Could you check a few things on this model? Use its own coordinates, in mm. Give positions to 0.01 mm unless a question says otherwise; leave off trailing zeros. Loops run counter-clockwise (first coordinate to the right, second up) from the corner with the lowest first, then second, coordinate; pieces in that order, holes last. Notation, with made-up numbers: (1.5, 21) - (52.5, 21) arc R21 ccw to (52.5, 57) - close; hole circle Ø7 at (-21, 12). An arc over 180 degrees is marked (long way). One line per item, written item: value. Start each with the question number.
Q1. I want a section at B-B (z = 10.25). Please give me the cut outline in (x, y).
Q2. I want a section at A-A (z = 3.25). Please give me the cut outline in (x, y), then the cut area to 3 significant figures.
Q3. If we mould it in two halves opening along Z, with no side actions, what happens to faces 1 (the face through (12, -39, 14)), 2 (the face through (40, -14, 5)), 3 (the face through (20, -39, 0))? For each: released by +Z, released by -Z, zero draft, split by the parting line, or undercut.
Q4. If I drill on line 1 (Y direction, x = 25, z = 8); line 2 (Y direction, x = 21, z = 9); line 3 (X direction, y = -7.5, z = 12.25), over which ranges is the centre line in solid material (lowest first)? Write a range as from..to.
```python
from build123d import *

# Parameters (mm, degrees)
F0_W         = 40
F0_H         = 80
F1_DEPTH     = 14
F4_T1_DEPTH  = 17.8405087492
F4_T3_DEPTH  = 17.8405087492
F4_T5_DEPTH  = 36
F4_T7_DEPTH  = 76
F4_T9_DEPTH  = 17
F4_S13_W     = 2
F4_S13_H     = 2
F4_T14_DEPTH = 2
F4_S19_W     = 2
F4_S19_H     = 2
F4_T20_DEPTH = 2
F4_S25_W     = 2
F4_S25_H     = 2
F4_T26_DEPTH = 2
F4_S31_W     = 2
F4_S31_H     = 2
F4_T32_DEPTH = 2
F4_T36_ANGLE = 193.2912055484


# Not quite as in the source:
# - a fillet or chamfer that OpenCascade refuses, or shapes differently, is made with other operations: its cross-section is extruded or revolved along the edge and cut away or added


with BuildPart() as f1:
    # F0 (on Top) → F1 (new body)
    with BuildSketch(Plane.XY):
        with Locations((20, -40)):
            Rectangle(F0_W, F0_H)
    extrude(amount=F1_DEPTH)

    # F2 (on face) → F3 (revolve, cut)
    with BuildSketch(Plane.YZ.offset(40)):
        with BuildLine():
            Line((-40, 0), (-32.5033340744, 0))
            ThreePointArc((-32.5033340744, 0), (-22.2346925053, 5.186748348), (-14.8405087492, 14))
            Line((-14.8405087492, 14), (-40, 14))
            Line((-40, 14), (-40, 0))
        make_face()
        with BuildLine():
            Line((-40, 14), (-14.8405087492, 14))
            ThreePointArc((-14.8405087492, 14), (-15.4345771459, 42.2458185159), (-40, 56.2))
            Line((-40, 56.2), (-40, 14))
        make_face()
        with BuildLine():
            Line((-40, 0), (-40, -1))
            ThreePointArc((-40, -1), (-36.2184659198, -0.7488976858), (-32.5033340744, 0))
            Line((-32.5033340744, 0), (-40, 0))
        make_face()
    revolve(axis=Axis((40, -40, 27.6), (0, 0, -1)), mode=Mode.SUBTRACT)

    # F4: fillet of radius 2 on 10 edges, made by hand

    # F4_s2 → F4_t1 (cut)
    with BuildSketch(Plane.XZ.offset(2)):
        with BuildLine():
            ThreePointArc((40, 12), (39.4142135624, 13.4142135624), (38, 14))
            Line((38, 14), (40, 14))
            Line((40, 14), (40, 12))
        make_face()
    extrude(amount=F4_T1_DEPTH, mode=Mode.SUBTRACT)

    # F4_s4 → F4_t3 (cut)
    with BuildSketch(Plane.XZ.offset(60.1594912508)):
        with BuildLine():
            ThreePointArc((38, 14), (39.4142135624, 13.4142135624), (40, 12))
            Line((40, 12), (40, 14))
            Line((40, 14), (38, 14))
        make_face()
    extrude(amount=F4_T3_DEPTH, mode=Mode.SUBTRACT)

    # F4_s6 → F4_t5 (cut)
    with BuildSketch(Plane.YZ.offset(2)):
        with BuildLine():
            ThreePointArc((-78, 14), (-79.4142135624, 13.4142135624), (-80, 12))
            Line((-80, 12), (-80, 14))
            Line((-80, 14), (-78, 14))
        make_face()
        with BuildLine():
            ThreePointArc((0, 12), (-0.5857864376, 13.4142135624), (-2, 14))
            Line((-2, 14), (0, 14))
            Line((0, 14), (0, 12))
        make_face()
    extrude(amount=F4_T5_DEPTH, mode=Mode.SUBTRACT)

    # F4_s8 → F4_t7 (cut)
    with BuildSketch(Plane.XZ.offset(2)):
        with BuildLine():
            ThreePointArc((0, 12), (0.5857864376, 13.4142135624), (2, 14))
            Line((2, 14), (0, 14))
            Line((0, 14), (0, 12))
        make_face()
    extrude(amount=F4_T7_DEPTH, mode=Mode.SUBTRACT)

    # F4_s10 → F4_t9 (cut)
    with BuildSketch(Plane.XY.offset(-5)):
        with BuildLine():
            ThreePointArc((38, -80), (39.4142135624, -79.4142135624), (40, -78))
            Line((40, -78), (40, -80))
            Line((40, -80), (38, -80))
        make_face()
        with BuildLine():
            ThreePointArc((0, -78), (0.5857864376, -79.4142135624), (2, -80))
            Line((2, -80), (0, -80))
            Line((0, -80), (0, -78))
        make_face()
        with BuildLine():
            ThreePointArc((38, 0), (39.4142135624, -0.5857864376), (40, -2))
            Line((40, -2), (40, 0))
            Line((40, 0), (38, 0))
        make_face()
        with BuildLine():
            ThreePointArc((2, 0), (0.5857864376, -0.5857864376), (0, -2))
            Line((0, -2), (0, 0))
            Line((0, 0), (2, 0))
        make_face()
    extrude(amount=F4_T9_DEPTH, mode=Mode.SUBTRACT)


with BuildPart() as f4_tool12:
    # F4_s13 → F4_t14 (new body)
    with BuildSketch(Plane.XZ.offset(2)):
        with Locations((39, 13)):
            Rectangle(F4_S13_W, F4_S13_H)
    extrude(amount=-F4_T14_DEPTH)

    # F4_s15 → F4_t16 (revolve, cut)
    with BuildSketch(Plane(origin=(38, -2, 12), x_dir=(-0.7071067812, 0, -0.7071067812), z_dir=(0.7071067812, 0, -0.7071067812))):
        with BuildLine():
            ThreePointArc((0, -2), (2, 0), (0, 2))
            Line((0, 2), (0, -2))
        make_face()
    revolve(axis=Axis((38, -2, 12), (0, 1, 0)), mode=Mode.SUBTRACT)


with BuildPart() as f1_1:
    add(f1.part)

    # F4_t11: cut F4_tool12
    add(f4_tool12.part, mode=Mode.SUBTRACT)


with BuildPart() as f4_tool18:
    # F4_s19 → F4_t20 (new body)
    with BuildSketch(Plane.XY.offset(12)):
        with Locations((39, -79)):
            Rectangle(F4_S19_W, F4_S19_H)
    extrude(amount=F4_T20_DEPTH)

    # F4_s21 → F4_t22 (revolve, cut)
    with BuildSketch(Plane(origin=(38, -78, 12), x_dir=(-0.7071067812, 0.7071067812, 0), z_dir=(0.7071067812, 0.7071067812, 0))):
        with BuildLine():
            ThreePointArc((0, -2), (2, 0), (0, 2))
            Line((0, 2), (0, -2))
        make_face()
    revolve(axis=Axis((38, -78, 12), (0, 0, 1)), mode=Mode.SUBTRACT)


with BuildPart() as f1_2:
    add(f1_1.part)

    # F4_t17: cut F4_tool18
    add(f4_tool18.part, mode=Mode.SUBTRACT)


with BuildPart() as f4_tool24:
    # F4_s25 → F4_t26 (new body)
    with BuildSketch(Plane.YZ.offset(2)):
        with Locations((-79, 13)):
            Rectangle(F4_S25_W, F4_S25_H)
    extrude(amount=-F4_T26_DEPTH)

    # F4_s27 → F4_t28 (revolve, cut)
    with BuildSketch(Plane(origin=(2, -78, 12), x_dir=(0, 0.7071067812, -0.7071067812), z_dir=(0, 0.7071067812, 0.7071067812))):
        with BuildLine():
            ThreePointArc((0, -2), (2, 0), (0, 2))
            Line((0, 2), (0, -2))
        make_face()
    revolve(axis=Axis((2, -78, 12), (-1, 0, 0)), mode=Mode.SUBTRACT)


with BuildPart() as f1_3:
    add(f1_2.part)

    # F4_t23: cut F4_tool24
    add(f4_tool24.part, mode=Mode.SUBTRACT)


with BuildPart() as f4_tool30:
    # F4_s31 → F4_t32 (new body)
    with BuildSketch(Plane.XZ.offset(2)):
        with Locations((1, 13)):
            Rectangle(F4_S31_W, F4_S31_H)
    extrude(amount=-F4_T32_DEPTH)

    # F4_s33 → F4_t34 (revolve, cut)
    with BuildSketch(Plane(origin=(2, -2, 12), x_dir=(0.7071067812, 0, -0.7071067812), z_dir=(0.7071067812, 0, 0.7071067812))):
        with BuildLine():
            ThreePointArc((0, -2), (2, 0), (0, 2))
            Line((0, 2), (0, -2))
        make_face()
    revolve(axis=Axis((2, -2, 12), (0, 1, 0)), mode=Mode.SUBTRACT)


with BuildPart() as f1_4:
    add(f1_3.part)

    # F4_t29: cut F4_tool30
    add(f4_tool30.part, mode=Mode.SUBTRACT)

    # F4_s35 → F4_t36 (revolve, cut)
    with BuildSketch(Plane(origin=(44.0622906263, -5.1337237407, 0), x_dir=(0, 0, 1), z_dir=(0.9932809704, -0.1157277578, 0))):
        with BuildLine():
            ThreePointArc((14, 8.7772353391), (13.7377018856, 9.7673828821), (13.0196078431, 10.4978165916))
            ThreePointArc((13.0196078431, 10.4978165916), (13.5070698024, 10.2153987353), (14, 9.9426372505))
            Line((14, 9.9426372505), (14, 8.7772353391))
        make_face()
    revolve(axis=Axis((40, -40, 14), (0, 0, 1)), revolution_arc=F4_T36_ANGLE, mode=Mode.SUBTRACT)


solid = f1_4.part
```
Worked answers:
1. outline: (0, -78) arc R2 ccw to (2, -80) - (38, -80) arc R2 ccw to (40, -78) - (40, -62.74) arc R22.74 cw to (40, -17.26) - (40, -2) arc R2 ccw to (38, 0) - (2, 0) arc R2 ccw to (0, -2) - close
2. outline: (0, -78) arc R2 ccw to (2, -80) - (38, -80) arc R2 ccw to (40, -78) - (40, -55) arc R15 cw to (40, -25) - (40, -2) arc R2 ccw to (38, 0) - (2, 0) arc R2 ccw to (0, -2) - close
2. area: 2,840 mm²
3. face 1: released by +Z
3. face 2: zero draft
3. face 3: released by -Z
4. line 1: y = -80..-54.45, -25.55..0
4. line 2: y = -80..-50.54, -29.46..0
4. line 3: x = 0.02..39.98
